```python
from build123d import *

# Parameters (mm, degrees)
MODEL_R             = 3.7
BOSS_EXTRUDE1_DEPTH = 800.5


with BuildPart() as part:
    # Model → Boss-Extrude1 (new body)
    with BuildSketch(Plane.XY):
        with BuildLine():
            Line((0.5, 8), (1.472732261, 8))
            ThreePointArc((1.472732261, 8), (4.799135414, 8.56946226), (7.746686356, 10.212991588))
            Line((7.746686356, 10.212991588), (10.25, 12.229898987))
            Line((10.25, 12.229898987), (10.25, 17))
            Line((10.25, 17), (5.1, 17))
            Line((5.1, 17), (5.1, 21))
            Line((5.1, 21), (5.999986755, 21))
            Line((5.999986755, 21), (5.999986755, 22.5))
            Line((5.999986755, 22.5), (22.5, 22.5))
            Line((22.5, 22.5), (22.5, 5.999986755))
            Line((22.5, 5.999986755), (21, 5.999986755))
            Line((21, 5.999986755), (21, 5.1))
            Line((21, 5.1), (17, 5.1))
            Line((17, 5.1), (17, 10.25))
            Line((17, 10.25), (12.229898987, 10.25))
            Line((12.229898987, 10.25), (10.212991588, 7.746686356))
            ThreePointArc((10.212991588, 7.746686356), (8.56946226, 4.799135414), (8, 1.472732261))
            Line((8, 1.472732261), (8, 0.5))
            Line((8, 0.5), (7.5, 0))
            Line((7.5, 0), (8, -0.5))
            Line((8, -0.5), (8, -1.472732261))
            ThreePointArc((8, -1.472732261), (8.56946226, -4.799135414), (10.212991588, -7.746686356))
            Line((10.212991588, -7.746686356), (12.229898987, -10.25))
            Line((12.229898987, -10.25), (17, -10.25))
            Line((17, -10.25), (17, -5.1))
            Line((17, -5.1), (21, -5.1))
            Line((21, -5.1), (21, -6.000013245))
            Line((21, -6.000013245), (22.5, -6.000013245))
            Line((22.5, -6.000013245), (22.5, -22.5))
            Line((22.5, -22.5), (6.000013245, -22.5))
            Line((6.000013245, -22.5), (6.000013245, -21))
            Line((6.000013245, -21), (5.1, -21))
            Line((5.1, -21), (5.1, -17))
            Line((5.1, -17), (10.25, -17))
            Line((10.25, -17), (10.25, -12.229898987))
            Line((10.25, -12.229898987), (7.746686356, -10.212991588))
            ThreePointArc((7.746686356, -10.212991588), (4.799135414, -8.56946226), (1.472732261, -8))
            Line((1.472732261, -8), (0.5, -8))
            Line((0.5, -8), (0, -7.5))
            Line((0, -7.5), (-0.5, -8))
            Line((-0.5, -8), (-1.472732261, -8))
            ThreePointArc((-1.472732261, -8), (-4.799135414, -8.56946226), (-7.746686356, -10.212991588))
            Line((-7.746686356, -10.212991588), (-10.25, -12.229898987))
            Line((-10.25, -12.229898987), (-10.25, -17))
            Line((-10.25, -17), (-5.1, -17))
            Line((-5.1, -17), (-5.1, -21))
            Line((-5.1, -21), (-5.999986755, -21))
            Line((-5.999986755, -21), (-5.999986755, -22.5))
            Line((-5.999986755, -22.5), (-22.5, -22.5))
            Line((-22.5, -22.5), (-22.5, -5.999986755))
            Line((-22.5, -5.999986755), (-21, -5.999986755))
            Line((-21, -5.999986755), (-21, -5.1))
            Line((-21, -5.1), (-17, -5.1))
            Line((-17, -5.1), (-17, -10.25))
            Line((-17, -10.25), (-12.229898987, -10.25))
            Line((-12.229898987, -10.25), (-10.212991588, -7.746686356))
            ThreePointArc((-10.212991588, -7.746686356), (-8.56946226, -4.799135414), (-8, -1.472732261))
            Line((-8, -1.472732261), (-8, -0.5))
            Line((-8, -0.5), (-7.5, 0))
            Line((-7.5, 0), (-8, 0.5))
            Line((-8, 0.5), (-8, 1.472732261))
            ThreePointArc((-8, 1.472732261), (-8.56946226, 4.799135414), (-10.212991588, 7.746686356))
            Line((-10.212991588, 7.746686356), (-12.229898987, 10.25))
            Line((-12.229898987, 10.25), (-17, 10.25))
            Line((-17, 10.25), (-17, 5.1))
            Line((-17, 5.1), (-21, 5.1))
            Line((-21, 5.1), (-21, 6.000013245))
            Line((-21, 6.000013245), (-22.5, 6.000013245))
            Line((-22.5, 6.000013245), (-22.5, 22.5))
            Line((-22.5, 22.5), (-6.000013245, 22.5))
            Line((-6.000013245, 22.5), (-6.000013245, 21))
            Line((-6.000013245, 21), (-5.1, 21))
            Line((-5.1, 21), (-5.1, 17))
            Line((-5.1, 17), (-10.25, 17))
            Line((-10.25, 17), (-10.25, 12.229898987))
            Line((-10.25, 12.229898987), (-7.746686356, 10.212991588))
            ThreePointArc((-7.746686356, 10.212991588), (-4.799135414, 8.56946226), (-1.472732261, 8))
            Line((-1.472732261, 8), (-0.5, 8))
            Line((-0.5, 8), (0, 7.5))
            Line((0, 7.5), (0.5, 8))
        make_face()
        Circle(MODEL_R, mode=Mode.SUBTRACT)
        Polygon((20.25, -9.25), (20.25, -20.25), (9.25, -20.25), (9.25, -18.75), (12.25, -18.75), (12.25, -12.25), (18.75, -12.25), (18.75, -9.25), align=None, mode=Mode.SUBTRACT)
        Polygon((9.25, 20.25), (20.25, 20.25), (20.25, 9.25), (18.75, 9.25), (18.75, 12.25), (12.25, 12.25), (12.25, 18.75), (9.25, 18.75), align=None, mode=Mode.SUBTRACT)
        Polygon((-9.25, -20.25), (-20.25, -20.25), (-20.25, -9.25), (-18.75, -9.25), (-18.75, -12.25), (-12.25, -12.25), (-12.25, -18.75), (-9.25, -18.75), align=None, mode=Mode.SUBTRACT)
        Polygon((-20.25, 20.25), (-9.25, 20.25), (-9.25, 18.75), (-12.25, 18.75), (-12.25, 12.25), (-18.75, 12.25), (-18.75, 9.25), (-20.25, 9.25), align=None, mode=Mode.SUBTRACT)
    extrude(amount=-BOSS_EXTRUDE1_DEPTH)


solid = part.part
```
The model under review builds one solid part; all positions refer to its coordinate system, in mm. Round coordinates to 2 decimals unless told otherwise and drop trailing zeros.
1) Consider section A-A on z = -321.5. Give the number of separate pieces and of enclosed holes in the cut face, then the cut area to 3 significant figures.
Values follow:
separate pieces: 1
enclosed holes: 5
area: 816 mm2
2) Clearance check with flat-ended pins moving along their axes: P1, Ø4, axis at x = -5, y = 11.5, coming from the -Z side; P2, Ø2, axis at y = 0.5, z = -424.5, coming from the +X side; P3, Ø0.5, axis at x = 1, z = -520.5, coming from the -Y side; P4, Ø1.5, axis at x = -4, z = -259.5, coming from the +Y side. State where each tip first meets the part, or that it passes through.
Values follow:
P1: passes through
P2: stops at x = 8
P3: stops at y = -8
P4: stops at y = 8.55
3) Wall thickness on line 1 along X through (y, z) = (14.5, -383); line 2 along Y through (x, z) = (-20, -110): over which ranges is each line inside the solid? List them lowest first.
Values follow:
line 1: x = -22.5 to -20.25, -12.25 to -10.25, 10.25 to 12.25, 20.25 to 22.5
line 2: y = -22.5 to -20.25, -9.25 to -5.1, 5.1 to 9.25, 20.25 to 22.5
